```python
from build123d import *

# Parameters (mm, degrees)
SKETCH1_W                                      = 100
SKETCH1_H                                      = 75
BOSS_EXTRUDE1_DEPTH                            = 4.5
CBORE_FOR_M3_SOCKET_HEAD_CAP_SCREW1_AT_2_COUNT = 2
CBORE_FOR_M3_SOCKET_HEAD_CAP_SCREW1_AT_2_PITCH = 56
CBORE_FOR_M3_SOCKET_HEAD_CAP_SCREW1_AT_3_COUNT = 2
CBORE_FOR_M3_SOCKET_HEAD_CAP_SCREW1_AT_3_PITCH = 84.876380696
CBORE_FOR_M3_SOCKET_HEAD_CAP_SCREW1_AT_4_COUNT = 2
CBORE_FOR_M3_SOCKET_HEAD_CAP_SCREW1_AT_4_PITCH = 70.455659815
SKETCH5_W                                      = 5
SKETCH5_H                                      = 75
BOSS_EXTRUDE2_DEPTH                            = 50
BOSS_EXTRUDE2_DEPTH_BACK                       = 4.5
SKETCH7_W                                      = 4.5
SKETCH7_H                                      = 12.1
BOSS_EXTRUDE3_DEPTH                            = 3.1
SKETCH6_R                                      = 1
SKETCH6_W                                      = 16.599006094
SKETCH6_H                                      = 12.1
CUT_EXTRUDE1_DEPTH                             = 10
CUT_EXTRUDE1_DEPTH_BACK                        = 9.1
SKETCH8_R                                      = 8.5
CUT_EXTRUDE2_DEPTH                             = 9.1


with BuildPart() as part:
    # Sketch1 → Boss-Extrude1 (new body)
    with BuildSketch(Plane(origin=(0, 0, 0), x_dir=(1, 0, 0), z_dir=(0, 1, 0))):
        with Locations((11.109271523, 14.701986755)):
            Rectangle(SKETCH1_W, SKETCH1_H)
    extrude(amount=BOSS_EXTRUDE1_DEPTH)

    # Sketch4 → CBORE for M3 Socket Head Cap Screw1 (revolve, cut)
    with BuildSketch(Plane(origin=(-23.219008058, 4.5, -42.701986755), x_dir=(0, 0, 1), z_dir=(1, 0, 0))):
        Polygon((0, 0), (0, 4.5), (1.7, 4.5), (1.7, 3), (3.25, 3), (3.25, 0.025), (3.275, 0), align=None)
    cbore_for_m3_socket_head_cap_screw1 = revolve(axis=Axis((-23.219008058, 10.85, -42.701986755), (0, -1, 0)), mode=Mode.SUBTRACT)

    # CBORE for M3 Socket Head Cap Screw1 at 2: CBORE for M3 Socket Head Cap Screw1 ×2
    with Locations(*[(0, 0, i * CBORE_FOR_M3_SOCKET_HEAD_CAP_SCREW1_AT_2_PITCH) for i in range(1, CBORE_FOR_M3_SOCKET_HEAD_CAP_SCREW1_AT_2_COUNT)]):
        add(cbore_for_m3_socket_head_cap_screw1, mode=Mode.SUBTRACT)

    # CBORE for M3 Socket Head Cap Screw1 at 3: CBORE for M3 Socket Head Cap Screw1 ×2
    with Locations(*[Vector(0.824728852, 0, 0.565528356) * (i * CBORE_FOR_M3_SOCKET_HEAD_CAP_SCREW1_AT_3_PITCH) for i in range(1, CBORE_FOR_M3_SOCKET_HEAD_CAP_SCREW1_AT_3_COUNT)]):
        add(cbore_for_m3_socket_head_cap_screw1, mode=Mode.SUBTRACT)

    # CBORE for M3 Socket Head Cap Screw1 at 4: CBORE for M3 Socket Head Cap Screw1 ×2
    with Locations(*[Vector(0.993532673, 0, 0.113546591) * (i * CBORE_FOR_M3_SOCKET_HEAD_CAP_SCREW1_AT_4_PITCH) for i in range(1, CBORE_FOR_M3_SOCKET_HEAD_CAP_SCREW1_AT_4_COUNT)]):
        add(cbore_for_m3_socket_head_cap_screw1, mode=Mode.SUBTRACT)

    # Sketch5 → Boss-Extrude2 (add, two sides)
    with BuildSketch(Plane(origin=(0, 4.5, 0), x_dir=(1, 0, 0), z_dir=(0, 1, 0))) as boss_extrude2_sk:
        with Locations((-41.390728477, 14.701986755)):
            Rectangle(SKETCH5_W, SKETCH5_H)
        with Locations((63.609271523, 14.701986755)):
            Rectangle(SKETCH5_W, SKETCH5_H)
    extrude(amount=BOSS_EXTRUDE2_DEPTH)
    extrude(boss_extrude2_sk.sketch, amount=-BOSS_EXTRUDE2_DEPTH_BACK)

    # Sketch7 → Boss-Extrude3 (add)
    with BuildSketch(Plane.ZY.offset(43.890728477)):
        with Locations((-28.701986755, 21.2)):
            Rectangle(SKETCH7_W, SKETCH7_H)
        with Locations((-0.701986755, 21.2)):
            Rectangle(SKETCH7_W, SKETCH7_H)
    extrude(amount=BOSS_EXTRUDE3_DEPTH)

    # Sketch6 → Cut-Extrude1 (cut, two sides)
    with BuildSketch(Plane.ZY.offset(43.890728477)) as cut_extrude1_sk:
        with Locations((-28.951986755, 21.2)):
            Circle(SKETCH6_R)
        with Locations((-0.451986755, 21.2)):
            Circle(SKETCH6_R)
        with Locations((-18.371105673, 21.2)):
            Rectangle(SKETCH6_W, SKETCH6_H)
    extrude(amount=CUT_EXTRUDE1_DEPTH, mode=Mode.SUBTRACT)
    extrude(cut_extrude1_sk.sketch, amount=-CUT_EXTRUDE1_DEPTH_BACK, mode=Mode.SUBTRACT)

    # Sketch8 → Cut-Extrude2 (cut)
    with BuildSketch(Plane(origin=(66.109271523, 0, 0), x_dir=(0, 0, -1), z_dir=(1, 0, 0))):
        with Locations((12.767684718, 25)):
            Circle(SKETCH8_R)
    extrude(amount=-CUT_EXTRUDE2_DEPTH, mode=Mode.SUBTRACT)


solid = part.part
```
The listing builds one solid part. Answer for the finished solid, in the listing's coordinates (mm). A direction names the side the tool comes from. Coordinates: 2 decimals unless noted, no trailing zeros. Write each loop counter-clockwise with the first axis right and the second up, starting at its lowest first coordinate (ties: lowest second). Pieces come first, ordered by that corner, then holes. Notation, with made-up numbers: M -38,89 L 10,89 A17 cw 10,105 Z; hole C 83,53.25 d3. An arc over 180 degrees is marked long. Use a Markdown table: item, result. Add a question column.
1. For a pull along X with two mould halves and no side action, classify faces 5 (the flat face through (-41, 21, -10.072)), 6 (the flat face through (-38.891, 29, -14)) as +X half, -X half, draft (parallel to the pull), parting line (faces both ways), or undercut.
2. Which of the six approach directions +Z, -Z, +X, -X, +Y, -Y give full straight-line access (tool end or side, diameter ignored) to faces 1 (the flat face through (48.2, 1.5, -36.1)), 2 (the flat face through (-45, 27.25, -1)), 3 (the flat face through (-45, 21, -2.952)), 4 (the flat face through (10, 4.5, -15))?
3. Section C-C (z = -8) is taken. Give the vertices of the cut face in (x, y), plus the area to 3 significant figures.
4. Section B-B (y = 46) is taken. Give the vertices of the cut face in (x, z), plus the area to 3 significant figures.
5. Straight lines are drawn through the part: line 1 along X through (y, z) = (16, 14.5); line 2 along X through (y, z) = (3, 13.5); line 3 along Y through (x, z) = (19.5, -34.5). For each, find the intervals that lie inside material, in ascending order. Write a range as [from, to].
6. Section A-A (y = 25) is taken. Give the vertices of the cut face in (x, z), plus the area to 3 significant figures.
7. Section D-D (x = 53) is taken. Give the vertices of the cut face in (y, z), plus the area to 4 significant figures.
8. Given P1, Ø3, axis at y = 48, z = -3, coming from the -X side; P2, Ø3, axis at x = 46.78, z = -34.7, coming from the -Y side; P3, Ø4, axis at x = 46.78, z = 5.3, coming from the +Y side; P4, Ø0.9, axis at x = -45, y = 20.5, coming from the +Z side, each flat-ended and moving along its own axis, determine where each tip first touches the part or whether it passes through.
Data:
| question | item | result |
|---|---|---|
| 1 | face 5 | draft |
| 1 | face 6 | undercut |
| 2 | face 1 | +Y |
| 2 | face 2 | +Z, -Z, -X, +Y |
| 2 | face 3 | -X, +Y, -Y |
| 2 | face 4 | +Z, -Z, +Y |
| 3 | outline | M -43.89,0 L 66.11,0 L 66.11,17.96 L 61.11,17.96 L 61.11,4.5 L -38.89,4.5 L -38.89,54.5 L -43.89,54.5 Z; M 61.11,32.04 L 66.11,32.04 L 66.11,54.5 L 61.11,54.5 Z |
| 3 | area | 925 mm2 |
| 4 | outline | M -43.89,-52.2 L -38.89,-52.2 L -38.89,22.8 L -43.89,22.8 Z; M 61.11,-52.2 L 66.11,-52.2 L 66.11,22.8 L 61.11,22.8 Z |
| 4 | area | 750 mm2 |
| 5 | line 1 | x = [-43.89, -38.89], [61.11, 66.11] |
| 5 | line 2 | x = [-43.89, -26.46], [-19.98, 66.11] |
| 5 | line 3 | y = [0, 4.5] |
| 6 | outline | M -46.99,-30.95 L -43.89,-30.95 L -43.89,-52.2 L -38.89,-52.2 L -38.89,-26.67 L -46.99,-26.67 Z; M -46.99,-2.95 L -43.89,-2.95 L -43.89,-10.07 L -38.89,-10.07 L -38.89,22.8 L -43.89,22.8 L -43.89,1.55 L -46.99,1.55 Z; M 61.11,-52.2 L 66.11,-52.2 L 66.11,-21.27 L 61.11,-21.27 Z; M 61.11,-4.27 L 66.11,-4.27 L 66.11,22.8 L 61.11,22.8 Z |
| 6 | area | 609 mm2 |
| 7 | outline | M 0,-52.2 L 4.5,-52.2 L 4.5,22.8 L 0,22.8 Z |
| 7 | area | 337.5 mm2 |
| 8 | P1 | stops at x = -43.89 |
| 8 | P2 | passes through |
| 8 | P3 | stops at y = 1.5 |
| 8 | P4 | stops at z = 1.55 |
